CAD build for the part. Positions are in the model's coordinates, mm. Round coordinates to 2 decimals unless told otherwise and drop trailing zeros. Loops run counter-clockwise (first coordinate to the right, second up) from the corner with the lowest first, then second, coordinate; pieces in that order, holes last.
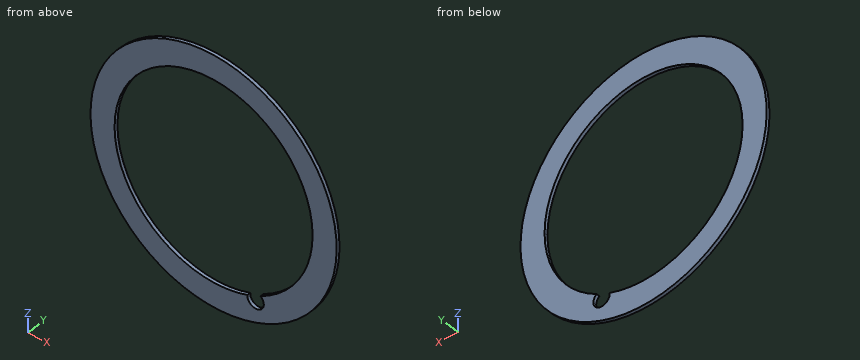
```python
from build123d import *

# Parameters (mm, degrees)
SKETCH1_R           = 142.875
BOSS_EXTRUDE2_DEPTH = 3.81


with BuildPart() as part:
    # Sketch1 → Boss-Extrude2 (new body)
    with BuildSketch(Plane(origin=(0, 0, 0), x_dir=(1, 0, 0), z_dir=(0, 1, 0))):
        with Locations(Location((0, 0, 0), (0, 0, 270))):
            Circle(SKETCH1_R)
        with BuildLine():
            ThreePointArc((54.490337546, 101.1971212), (98.67345431, 58.937285648), (114.935, 0))
            ThreePointArc((114.935, 0), (-94.142770704, -65.933246159), (39.288887865, 108.011284204))
            ThreePointArc((39.288887865, 108.011284204), (48.374639999, 118.336615411), (58.304474981, 108.820222521))
            ThreePointArc((58.304474981, 108.820222521), (57.297737448, 104.558200756), (54.490337546, 101.1971212))
        make_face(mode=Mode.SUBTRACT)
    extrude(amount=-BOSS_EXTRUDE2_DEPTH)


solid = part.part
```
Item 1: Flat gauge pins, fed straight in: P1, Ø1.5, axis at y = -3, z = -44.5, coming from the +X side; P2, Ø1, axis at y = -0.5, z = -46.5, coming from the +X side. Where does each tip first touch, or does it go through?
Answers follow:
P1: stops at x = 136.01
P2: stops at x = 135.27
Item 2: Probe line 1 (X direction, y = -2.55, z = 0) (3 decimals); line 2 (X direction, y = -2.95, z = -94); line 3 (Z direction, x = 41.5, y = -1.6). List the from-to ranges inside material, lowest first.
Answers follow:
line 1: x = -142.875 to -114.935, 114.935 to 142.875
line 2: x = -107.6 to -66.14, 66.14 to 107.6
line 3: z = -136.72 to -114.96, 107.18 to 136.72
Item 3: Cut at B-B, the plane z = 5.5. Give the cut face in (x, y), plus the area to 3 significant figures.
Answers follow:
outline: (-142.77, -3.81) - (-114.8, -3.81) - (-114.8, 0) - (-142.77, 0) - close; (114.8, -3.81) - (142.77, -3.81) - (142.77, 0) - (114.8, 0) - close
area: 213 mm2
Item 4: Cut at D-D, the plane z = -125. Give the cut face in (x, y).
Answers follow:
outline: (-69.2, -3.81) - (69.2, -3.81) - (69.2, 0) - (-69.2, 0) - close
Item 5: Cut at A-A, the plane x = 0. Give the cut face in (y, z) (3 decimals).
Answers follow:
outline: (-3.81, -142.875) - (0, -142.875) - (0, -114.935) - (-3.81, -114.935) - close; (-3.81, 114.935) - (0, 114.935) - (0, 142.875) - (-3.81, 142.875) - close
Item 6: Cut at C-C, the plane y = -1.15. Give the cut face in (x, z) (3 decimals), plus the area to 3 significant figures.
Answers follow:
outline: circle Ø285.75 at (0, 0); hole (39.289, -108.011) arc R9.525 ccw (long way) to (54.49, -101.197) arc R114.935 ccw (long way) to start
area: 22,400 mm2
